The listing builds one solid part. Answer for the finished solid, in the listing's coordinates (mm). A direction names the side the tool comes from. Round coordinates to 2 decimals unless told otherwise and drop trailing zeros. Order: outer loops, then holes, each group sorted by start corner. A loop starts at its lowest first (then second) coordinate and runs counter-clockwise, first axis right, second up. Notation, with made-up numbers: (5, -5.5) - (13, -5.5) arc R13 ccw to (13, -0.5) - close; hole circle Ø10 at (-12.75, 14). An arc over 180 degrees is marked (long way). Write item = value, one per line.
from build123d import *

# Parameters (mm, degrees)
CYLINDER009_R     = 18.5
CYLINDER009_DEPTH = 1.5
CYLINDER008_R     = 31
CYLINDER008_DEPTH = 1.5
CYLINDER007_R     = 27.5
CYLINDER007_DEPTH = 10
CYLINDER006_R     = 27.5
CYLINDER006_DEPTH = 1.5
CYLINDER005_R     = 29.5
CYLINDER005_DEPTH = 1.5


with BuildPart() as cone002:
    # Cone002 → Cone002 (revolve)
    with BuildSketch(Plane.XZ):
        Polygon((0, 0), (29, 0), (60, 40), (0, 40), align=None)
    revolve(axis=Axis((0, 0, 0), (0, 0, 1)))


with BuildPart() as cut013:
    # Cone003 → Cone003 (revolve)
    with BuildSketch(Plane.XZ):
        Polygon((0, 0), (31, 0), (62, 40), (0, 40), align=None)
    revolve(axis=Axis((0, 0, 0), (0, 0, 1)))

    # Cut013: cut Cone002
    add(cone002.part, mode=Mode.SUBTRACT)


with BuildPart() as cut013_1:
    # Cut013 placement: moved
    add(cut013.part.moved(Location((83, 32, 99.5))))


with BuildPart() as cylinder009:
    # Cylinder009 → Cylinder009 (new body)
    with BuildSketch(Plane.XY):
        Circle(CYLINDER009_R)
    extrude(amount=CYLINDER009_DEPTH)


with BuildPart() as cut010:
    # Cylinder008 → Cylinder008 (new body)
    with BuildSketch(Plane.XY):
        Circle(CYLINDER008_R)
    extrude(amount=CYLINDER008_DEPTH)

    # Cut010: cut Cylinder009
    add(cylinder009.part, mode=Mode.SUBTRACT)


with BuildPart() as cut010_1:
    # Cut010 placement: moved
    add(cut010.part.moved(Location((0, 0, 1.5))))


with BuildPart() as cylinder007:
    # Cylinder007 → Cylinder007 (new body)
    with BuildSketch(Plane.XY):
        Circle(CYLINDER007_R)
    extrude(amount=CYLINDER007_DEPTH)


with BuildPart() as cylinder006:
    # Cylinder006 → Cylinder006 (new body)
    with BuildSketch(Plane.XY):
        Circle(CYLINDER006_R)
    extrude(amount=CYLINDER006_DEPTH)


with BuildPart() as union:
    # Cylinder005 → Cylinder005 (new body)
    with BuildSketch(Plane.XY):
        Circle(CYLINDER005_R)
    extrude(amount=CYLINDER005_DEPTH)

    # Cut008: cut Cylinder006
    add(cylinder006.part, mode=Mode.SUBTRACT)

    # Cut009: cut Cylinder007
    add(cylinder007.part, mode=Mode.SUBTRACT)

    # Fusion004: union Cut010
    add(cut010_1.part)


with BuildPart() as union_1:
    # Fusion004 placement: moved
    add(union.part.moved(Location((83, 32, 98.5))))

    # Cut014: cut Cut013
    add(cut013_1.part, mode=Mode.SUBTRACT)


solid = union_1.part
Q1. Section C-C on z = 100.7 is taken. Determine the outline of the cut face in (x, y).
Model answer:
outline = circle Ø59.86 at (83, 32); hole circle Ø37 at (83, 32)
Q2. Section B-B on x = 83 is taken. Determine the outline of the cut face in (y, z), then the cut area to 3 significant figures.
Model answer:
outline = (1.45, 101.5) - (3, 99.5) - (2.5, 99.5) - (2.5, 98.5) - (4.5, 98.5) - (4.5, 100) - (13.5, 100) - (13.5, 101.5) - close; (50.5, 100) - (59.5, 100) - (59.5, 98.5) - (61.5, 98.5) - (61.5, 99.5) - (61, 99.5) - (62.55, 101.5) - (50.5, 101.5) - close
area = 40.1 mm^2
Q3. Section A-A on y = 32 is taken. Determine the outline of the cut face in (x, z).
Model answer:
outline = (52.45, 101.5) - (54, 99.5) - (53.5, 99.5) - (53.5, 98.5) - (55.5, 98.5) - (55.5, 100) - (64.5, 100) - (64.5, 101.5) - close; (101.5, 100) - (110.5, 100) - (110.5, 98.5) - (112.5, 98.5) - (112.5, 99.5) - (112, 99.5) - (113.55, 101.5) - (101.5, 101.5) - close
Q4. Determine the mould class of faces 4 (the face through (68.32, 20.74, 100.74)), 5 (the face through (96.2, 18.8, 101.5)), 6 (the face through (110.25, 20.7, 98.99)) for opening direction X: released by +X, released by -X, zero draft, split by the parting line, or undercut.
Model answer:
face_4 = undercut
face_5 = zero draft
face_6 = split by the parting line
Q5. For faces 1 (the face through (101, 26, 100)), 2 (the face through (103, 12, 98.5)), 3 (the face through (61.29, 12.47, 99.5)), determine the directions among +Z, -Z, +X, -X, +Y, -Y from which every point of the face is accessible in a straight line to the end or side of a thin tool.
Model answer:
face_1 = -Z
face_2 = -Z, +X, -X, +Y, -Y
face_3 = none
Q6. Flat-ended cylindrical pins translate along their axes: P1, Ø1.5, axis at y = 15, z = 99.5, coming from the -X side; P2, Ø5, axis at x = 81.5, y = 51.5, coming from the -Z side; P3, Ø1.5, axis at y = 19, z = 100.5, coming from the +X side. Find the tip coordinate at first contact, or state that the pin passes through.
Model answer:
P1 = 58.38
P2 = 100
P3 = 110.52
Q7. Find the intervals of material crossed by line 1 (Y direction, x = 83, z = 98.85); line 2 (Y direction, x = 61.5, z = 98.7); line 3 (X direction, y = 39, z = 100.55), in increasing order. Write a range as from..to.
Model answer:
line_1 = 2.5..4.5, 59.5..61.5
line_2 = 11.8..14.85, 49.15..52.2
line_3 = 54.02..65.88, 100.12..111.98
